Read the model definition and answer for the solid it produces. Units are mm, in the model's axes. A direction names the side the tool comes from. Give positions to 0.01 mm unless a question says otherwise; leave off trailing zeros. Write each loop counter-clockwise with the first axis right and the second up, starting at its lowest first coordinate (ties: lowest second). Pieces come first, ordered by that corner, then holes. Notation, with made-up numbers: (27, 76.5) - (60, 76.5) arc R21 ccw to (60, 104.5) - close; hole circle Ø9 at (74.5, 52.25). An arc over 180 degrees is marked (long way). Answer as a JSON object with one key per item and string values. Group by question number.
```python
from build123d import *

# Parameters (mm, degrees)
SKETCH_1_R      = 1.65
EXTRUDE_1_DEPTH = 4
EXTRUDE_2_DEPTH = 30
FILLET_1_R      = 1
FILLET_2_R      = 1


with BuildPart() as part:
    # 草图1 → 凸台-拉伸1 (new body)
    with BuildSketch(Plane(origin=(0, 0, 0), x_dir=(1, 0, 0), z_dir=(0, 1, 0))):
        Polygon((-71.5, 3), (-71.5, -3), (-52.5, -3), (-46.5, 3), (46.5, 3), (52.5, -3), (71.5, -3), (71.5, 3), (53.5, 3), (51.5, 5), (-51.5, 5), (-53.5, 3), align=None)
        with Locations(Location((-57.5, 0, 0), (0, 0, 270))):
            Circle(SKETCH_1_R, mode=Mode.SUBTRACT)
        with Locations(Location((-67.5, 0, 0), (0, 0, 270))):
            Circle(SKETCH_1_R, mode=Mode.SUBTRACT)
        with Locations(Location((67.5, 0, 0), (0, 0, 90))):
            Circle(SKETCH_1_R, mode=Mode.SUBTRACT)
        with Locations(Location((57.5, 0, 0), (0, 0, 90))):
            Circle(SKETCH_1_R, mode=Mode.SUBTRACT)
    extrude(amount=EXTRUDE_1_DEPTH)

    # 草图2 → 凸台-拉伸2 (add)
    with BuildSketch(Plane(origin=(0, 4, 0), x_dir=(1, 0, 0), z_dir=(0, 1, 0))):
        Polygon((-51.5, 5), (-53.5, 3), (53.5, 3), (51.5, 5), align=None)
    extrude(amount=EXTRUDE_2_DEPTH)

    # 圆角1
    fillet_1_edges = [part.edges().sort_by_distance(p)[0] for p in [
        (51.5, 17, -5),
        (-51.5, 17, -5),
        (-71.5, 2, -3),
        (-71.5, 2, 3),
        (-46.5, 2, -3),
        (46.5, 2, -3),
        (52.5, 2, 3),
        (71.5, 2, 3),
        (71.5, 2, -3),
        (-52.5, 2, 3),
        (-53.5, 19, -3),
        (53.5, 19, -3),
    ]]
    fillet(fillet_1_edges, radius=FILLET_1_R - 0.0001)  # a hair under: the kernel refuses the full size

    # 圆角2
    fillet_2_edges = [part.edges().sort_by_distance(p)[0] for p in [
        (53.5, 2, -3),
        (-53.5, 2, -3),
    ]]
    fillet(fillet_2_edges, radius=FILLET_2_R)


solid = part.part
```
1) For a pull along X with two mould halves and no side action, classify faces 5 (the flat face through (-49.5, 2, 0)), 6 (the flat face through (-1, 0, -4)), 7 (the flat face through (71.5, 2, 0)) as released by +X, released by -X, zero draft, split by the parting line, or undercut.
2) Find section D-D, the plane x = -38.5. Write down the section's boundary in (y, z).
3) Find the intervals of material crossed by line 1 (Z direction, x = -67.5, y = 1.8); line 2 (Z direction, x = 12, y = 10); line 3 (Y direction, x = -51.5, z = -1.5), in increasing order. Write a range as [from, to].
4) Find section A-A, the plane z = 0. Write down the section's boundary in (x, y), and give its area (3 significant figures).
5) Flat-ended cylindrical pins translate along their axes: pin 1 Ø2 at (x, y) = (-63.5, 3) entering from -Z; pin 2 Ø17 at (x, y) = (-23, 10.5) entering from +Z; pin 3 Ø2.5 at (x, z) = (-59, -2.5) entering from +Y. Find the tip coordinate at first contact, or state that the pin passes through.
6) Which of the six approach directions +Z, -Z, +X, -X, +Y, -Y give full straight-line access (tool end or side, diameter ignored) to faces 1 (the flat face through (62, 2, -3)), 2 (the flat face through (49.5, 2, 0)), 3 (the flat face through (-62, 2, -3)), 4 (the flat face through (-62, 2, 3))?
7) Find section B-B, the plane x = 67.5. Write down the section's boundary in (y, z).
Values follow:
{
 "1": {"face 5": "undercut", "face 6": "zero draft", "face 7": "released by +X"},
 "2": {"outline": "(0, -5) - (34, -5) - (34, -3) - (0, -3) - close"},
 "3": {"line 1": "z = [-3, -1.65], [1.65, 3]", "line 2": "z = [-5, -3]", "line 3": "y = [0, 4]"},
 "4": {"outline": "(-71.5, 0) - (-69.15, 0) - (-69.15, 4) - (-71.5, 4) - close; (-65.85, 0) - (-59.15, 0) - (-59.15, 4) - (-65.85, 4) - close; (-55.85, 0) - (-49.5, 0) - (-49.5, 4) - (-55.85, 4) - close; (49.5, 0) - (55.85, 0) - (55.85, 4) - (49.5, 4) - close; (59.15, 0) - (65.85, 0) - (65.85, 4) - (59.15, 4) - close; (69.15, 0) - (71.5, 0) - (71.5, 4) - (69.15, 4) - close", "area": "123 mm2"},
 "5": {"pin 1": "stops at z = -3", "pin 2": "stops at z = -3", "pin 3": "stops at y = 4"},
 "6": {"face 1": "-Z, +X, +Y, -Y", "face 2": "+Z, +Y, -Y", "face 3": "-Z, -X, +Y, -Y", "face 4": "+Z, +X, -X, +Y, -Y"},
 "7": {"outline": "(0, -3) - (4, -3) - (4, -1.65) - (0, -1.65) - close; (0, 1.65) - (4, 1.65) - (4, 3) - (0, 3) - close"}
}
